Could you check a few things on this model? Use its own coordinates, in mm. A direction names the side the tool comes from. Coordinates: 2 decimals unless noted, no trailing zeros. Order: outer loops, then holes, each group sorted by start corner. A loop starts at its lowest first (then second) coordinate and runs counter-clockwise, first axis right, second up. Notation, with made-up numbers: (41, 82.25) - (83, 82.25) arc R22 cw to (83, 102.25) - close; hole circle Ø11 at (83.5, 76). An arc over 180 degrees is marked (long way). Answer as CSV lines item,"result". Start each with the question number.
1. I want a section at B-B, the plane y = 0. Count the separate pieces of the cut face and the enclosed holes in it, and give its area (3 significant figures).
2. I want a section at A-A, the plane x = 114. List the corners of the cut face in (y, z) for me, and give its area (3 significant figures).
3. For faces 1 (the face through (160, 0, -5)), 2 (the face through (160, 0, 4)), which set-ups out of +Z, -Z, +X, -X, +Y, -Y let a thin tool reach every point of the face, with its end or its side?
4. I need wall thicknesses on probe 1 along X at (y, z) = (4.55, 0); probe 2 along Y at (x, z) = (111, 3.25). Which ranges of each line are inside material? Lowest first, please.
5. For pin 1 (5 mm diameter, centred on x = 35, z = 0, fed in from +Y); pin 2 (2.5 mm diameter, centred on x = 22.5, y = 0, fed in from +Z), each with a flat end and sliding along its axis, tell me the tip position at first contact or that it passes through.
from build123d import *

# Parameters (mm, degrees)
SKETCH_1_W          = 10
SKETCH_1_H          = 10
SKETCH_1_W_2        = 8
SKETCH_1_H_2        = 8
EXTRUDE_1_DEPTH     = 325
SKETCH_2_R          = 2.1
CUT_EXTRUDE_1_DEPTH = 326.19225083
SKETCH_3_R          = 2.1
CUT_EXTRUDE_2_DEPTH = 326.19225083


with BuildPart() as part:
    # ｽｹｯﾁ1 → 押し出し-薄板1 (new body)
    with BuildSketch(Plane(origin=(0, 0, 0), x_dir=(0, 0, -1), z_dir=(1, 0, 0))):
        Rectangle(SKETCH_1_W, SKETCH_1_H)
        Rectangle(SKETCH_1_W_2, SKETCH_1_H_2, mode=Mode.SUBTRACT)
    extrude(amount=EXTRUDE_1_DEPTH)

    # ｽｹｯﾁ2 → ｶｯﾄ - 押し出し1 (cut, through all)
    with BuildSketch(Plane.XY.offset(5)):
        with Locations((22.5, 0)):
            Circle(SKETCH_2_R)
        with Locations((7.5, 0)):
            Circle(SKETCH_2_R)
        with Locations(Location((317.5, 0, 0), (0, 0, 90))):
            Circle(SKETCH_2_R)
        with Locations(Location((302.5, 0, 0), (0, 0, 90))):
            Circle(SKETCH_2_R)
    extrude(amount=-CUT_EXTRUDE_1_DEPTH, mode=Mode.SUBTRACT)

    # ｽｹｯﾁ3 → ｶｯﾄ - 押し出し2 (cut, through all)
    with BuildSketch(Plane(origin=(0, 5, 0), x_dir=(1, 0, 0), z_dir=(0, 1, 0))):
        with Locations(Location((275, 0, 0), (0, 0, 270))):
            Circle(SKETCH_3_R)
        with Locations(Location((290, 0, 0), (0, 0, 270))):
            Circle(SKETCH_3_R)
        with Locations(Location((35, 0, 0), (0, 0, 270))):
            Circle(SKETCH_3_R)
        with Locations(Location((50, 0, 0), (0, 0, 270))):
            Circle(SKETCH_3_R)
    extrude(amount=-CUT_EXTRUDE_2_DEPTH, mode=Mode.SUBTRACT)


solid = part.part
Solved:
1,separate pieces,"10"
1,enclosed holes,"0"
1,area,"616 mm2"
2,outline,"(-5, -5) - (5, -5) - (5, 5) - (-5, 5) - close; hole (-4, -4) - (4, -4) - (4, 4) - (-4, 4) - close"
2,area,"36.0 mm2"
3,face 1,"-Z, +X, -X, +Y, -Y"
3,face 2,"+X, -X"
4,probe 1,"x = 0 to 32.9, 37.1 to 47.9, 52.1 to 272.9, 277.1 to 287.9, 292.1 to 325"
4,probe 2,"y = -5 to -4, 4 to 5"
5,pin 1,"stops at y = 5"
5,pin 2,"passes through"
